from build123d import *

# Parameters (mm, degrees)
BOSS_EXTRUDE1_DEPTH = 36
CUT_EXTRUDE1_REACH  = 77.774
SKETCH5_W           = 10
SKETCH5_H           = 10
CUT_EXTRUDE4_DEPTH  = 70.808427336
SKETCH6_W           = 10
SKETCH6_H           = 49.869122111
CUT_EXTRUDE5_DEPTH  = 8.383745
SKETCH7_R           = 1.5
BOSS_EXTRUDE2_DEPTH = 10
BOSS_EXTRUDE3_DEPTH = 6
SKETCH9_R           = 5
BOSS_EXTRUDE4_DEPTH = 20.4
CUT_EXTRUDE7_REACH  = 76.44
SKETCH12_R          = 2
FILLET1_R           = 1.5


with BuildPart() as part:
    # Sketch1 → Boss-Extrude1 (new body)
    with BuildSketch(Plane.XY):
        Polygon((0, 0), (-26, 0), (-26, 10), (1.005154776, 56), (15.005154776, 56), align=None)
    extrude(amount=BOSS_EXTRUDE1_DEPTH)

    # Sketch2 → Cut-Extrude1 (cut, up to next)
    with BuildSketch(Plane(origin=(-26, 3.422964937, 0), x_dir=(0, 0, -1), z_dir=(1, 0, 0)), mode=Mode.PRIVATE) as cut_extrude1_sk1:
        with BuildLine():
            Line((-26, 36.577035063), (-26, 52.577035063))
            Line((-26, 52.577035063), (-36, 52.577035063))
            Line((-36, 52.577035063), (-36, 6.577035063))
            ThreePointArc((-36, 6.577035063), (-28.565835097, 20.765646762), (-26, 36.577035063))
        make_face()
    cut_extrude1_tool1 = extrude(cut_extrude1_sk1.sketch, amount=CUT_EXTRUDE1_REACH, mode=Mode.PRIVATE) & part.part
    # Sketch2 → Cut-Extrude1 (cut, up to next)
    with BuildSketch(Plane(origin=(-26, 3.422964937, 0), x_dir=(0, 0, -1), z_dir=(1, 0, 0)), mode=Mode.PRIVATE) as cut_extrude1_sk2:
        with BuildLine():
            ThreePointArc((-10, 36.577035063), (-7.434164903, 20.765646762), (0, 6.577035063))
            Line((0, 6.577035063), (0, 52.577035063))
            Line((0, 52.577035063), (-10, 52.577035063))
            Line((-10, 52.577035063), (-10, 36.577035063))
        make_face()
    cut_extrude1_tool2 = extrude(cut_extrude1_sk2.sketch, amount=CUT_EXTRUDE1_REACH, mode=Mode.PRIVATE) & part.part
    # Sketch2 → Cut-Extrude1 (cut, up to next)
    with BuildSketch(Plane(origin=(-26, 3.422964937, 0), x_dir=(0, 0, -1), z_dir=(1, 0, 0)), mode=Mode.PRIVATE) as cut_extrude1_sk3:
        with BuildLine():
            ThreePointArc((-36, 6.577035063), (-28.565835097, 20.765646762), (-26, 36.577035063))
            Line((-26, 36.577035063), (-26, 52.577035063))
            Line((-26, 52.577035063), (-36, 52.577035063))
            Line((-36, 52.577035063), (-36, 6.577035063))
        make_face()
    cut_extrude1_tool3 = extrude(cut_extrude1_sk3.sketch, amount=CUT_EXTRUDE1_REACH, mode=Mode.PRIVATE) & part.part
    # Sketch2 → Cut-Extrude1 (cut, up to next)
    with BuildSketch(Plane(origin=(-26, 3.422964937, 0), x_dir=(0, 0, -1), z_dir=(1, 0, 0)), mode=Mode.PRIVATE) as cut_extrude1_sk4:
        with BuildLine():
            Line((0, 6.577035063), (0, 52.577035063))
            Line((0, 52.577035063), (-10, 52.577035063))
            Line((-10, 52.577035063), (-10, 36.577035063))
            ThreePointArc((-10, 36.577035063), (-7.434164903, 20.765646762), (0, 6.577035063))
        make_face()
    cut_extrude1_tool4 = extrude(cut_extrude1_sk4.sketch, amount=CUT_EXTRUDE1_REACH, mode=Mode.PRIVATE) & part.part
    add(cut_extrude1_tool1.solids().sort_by_distance((-26, 37.109216, 31.540478))[0], mode=Mode.SUBTRACT)
    add(cut_extrude1_tool2.solids().sort_by_distance((-26, 37.109216, 4.459522))[0], mode=Mode.SUBTRACT)
    add(cut_extrude1_tool3.solids().sort_by_distance((-26, 37.109216, 31.540478))[0], mode=Mode.SUBTRACT)
    add(cut_extrude1_tool4.solids().sort_by_distance((-26, 37.109216, 4.459522))[0], mode=Mode.SUBTRACT)

    # Sketch5 → Cut-Extrude4 (cut, through all)
    with BuildSketch(Plane.ZY.offset(6)):
        with Locations((31, 5)):
            Rectangle(SKETCH5_W, SKETCH5_H)
        with Locations((5, 5)):
            Rectangle(SKETCH5_W, SKETCH5_H)
    extrude(amount=-CUT_EXTRUDE4_DEPTH, mode=Mode.SUBTRACT)

    # Sketch6 → Cut-Extrude5 (cut)
    with BuildSketch(Plane(origin=(0, 0, 0), x_dir=(0, 0, -1), z_dir=(0.9659258262890674, -0.2588190451025246, 0))):
        with Locations((-31, 33.040905048)):
            Rectangle(SKETCH6_W, SKETCH6_H)
        with Locations((-5, 33.040905048)):
            Rectangle(SKETCH6_W, SKETCH6_H)
    extrude(amount=-CUT_EXTRUDE5_DEPTH, mode=Mode.SUBTRACT)

    # Sketch7 → Boss-Extrude2 (add)
    with BuildSketch(Plane.XZ):
        Polygon((-26, 24), (-33, 34), (-33, 42), (-24, 42), (-24, 36), (-26, 36), align=None)
        with Locations(Location((-29.5, 37.5, 0), (0, 0, 270))):
            Circle(SKETCH7_R, mode=Mode.SUBTRACT)
        Polygon((-26, 0), (-24, 0), (-24, -6), (-33, -6), (-33, 2), (-26, 12), align=None)
        with Locations(Location((-29.5, -1.5, 0), (0, 0, 90))):
            Circle(SKETCH7_R, mode=Mode.SUBTRACT)
        Polygon((-6, 12), (1, 2), (1, -6), (-8, -6), (-8, 0), (-6, 0), align=None)
        with Locations(Location((-2.5, -1.5, 0), (0, 0, 270))):
            Circle(SKETCH7_R, mode=Mode.SUBTRACT)
        Polygon((-6, 36), (-8, 36), (-8, 42), (1, 42), (1, 34), (-6, 24), align=None)
        with Locations(Location((-2.5, 37.5, 0), (0, 0, 90))):
            Circle(SKETCH7_R, mode=Mode.SUBTRACT)
    extrude(amount=-BOSS_EXTRUDE2_DEPTH)

    # Sketch8 → Boss-Extrude3 (add, symmetric)
    with BuildSketch(Plane.XY.offset(18)):
        Polygon((-26, 5), (-26, 10), (0, 54.287840966), (0, 55.819136666), (-2, 55.819136666), (-27.5, 12.382984949), align=None)
    extrude(amount=BOSS_EXTRUDE3_DEPTH, both=True)

    # Sketch9 → Boss-Extrude4 (add)
    with BuildSketch(Plane(origin=(0, 0, 0), x_dir=(0, 0, -1), z_dir=(-0.9659258262890674, 0.2588190451025246, 0))):
        with Locations(Location((-18, -44.351999472, 0), (0, 0, 270))):
            Circle(SKETCH9_R)
    extrude(amount=BOSS_EXTRUDE4_DEPTH)

    # Sketch12 → Cut-Extrude7 (cut, up to next)
    with BuildSketch(Plane(origin=(-19.704886856, 5.27990852, 0), x_dir=(0, 0, 1), z_dir=(-0.9659258262890673, 0.2588190451025247, 0)), mode=Mode.PRIVATE) as cut_extrude7_sk1:
        with Locations(Location((18, 44.351999472, 0), (0, 0, 270))):
            Circle(SKETCH12_R)
    cut_extrude7_tool1 = extrude(cut_extrude7_sk1.sketch, amount=-CUT_EXTRUDE7_REACH, mode=Mode.PRIVATE) & part.part
    add(cut_extrude7_tool1.solids().sort_by_distance((-8.225745, 48.12065, 18))[0], mode=Mode.SUBTRACT)

    # Fillet1
    fillet1_edges = [part.edges().sort_by_distance(p)[0] for p in [
        (-28.5, 10, 42),
        (-28.5, 10, -6),
        (-3.5, 10, -6),
        (-3.5, 10, 42),
    ]]
    fillet(fillet1_edges, radius=FILLET1_R)


solid = part.part
Read the model definition and answer for the solid it produces. Units are mm, in the model's axes. A direction names the side the tool comes from. Round coordinates to 2 decimals unless told otherwise and drop trailing zeros. Order: outer loops, then holes, each group sorted by start corner. A loop starts at its lowest first (then second) coordinate and runs counter-clockwise, first axis right, second up.
1) Straight lines are drawn through the part: L1, parallel to X at y = 5.5, z = -1.5; L2, parallel to Z at x = -29, y = 6; L3, parallel to Z at x = -2, y = 4. For each, find the intervals that lie inside material, in ascending order.
2) Flat-ended cylindrical pins translate along their axes: pin 1 (2.5 mm diameter, centred on x = -2.5, z = 37.5, fed in from -Y); pin 2 (3 mm diameter, centred on x = -12, y = 12, fed in from +Z); pin 3 (4 mm diameter, centred on x = -20.5, z = 22.5, fed in from +Y); pin 4 (6.5 mm diameter, centred on y = 4, z = -1, fed in from +X). Find the tip coordinate at first contact, or state that the pin passes through.
3) For faces 1 (the face through (-1.84, 4.93, 6.06)), 2 (the face through (-26.76, 8.74, 18.08)), 3 (the face through (-28.44, 9.55, 41.57)), 4 (the face through (-28, 10, 2)), determine the directions among +Z, -Z, +X, -X, +Y, -Y from which every point of the face is accessible in a straight line to the end or side of a thin tool.
4) The part is cut by section A-A on x = -29.5. Write down the section's boundary in (y, z), plus the area to 3 significant figures.
5) The part is cut by section C-C on y = 7. Write down the section's boundary in (x, z).
6) The mould has two halves that part along Y. Classify faces 5 (the face through (-5.88, 52.43, 16.5)), 6 (the face through (-16, 5, 36)), 7 (the face through (-3.56, 9.57, -5.55)): released by +Y, released by -Y, zero draft, split by the parting line, or undercut.
7) The part is cut by section B-B on z = -1.5. Write down the section's boundary in (x, y).
8) The part is cut by section D-D on x = -22. Write down the section's boundary in (y, z).
Resolved:
1. L1: x = -33 to -31, -28 to -24, -8 to -4, -1 to 1
1. L2: z = -6 to -2.91, -0.09 to 7.71, 28.29 to 36.09, 38.91 to 42
1. L3: z = -6 to -2.91, -0.09 to 6.29, 10 to 26, 29.71 to 36.09, 38.91 to 42
2. pin 1: passes through
2. pin 2: stops at z = 35.63
2. pin 3: stops at y = 27.71
2. pin 4: stops at x = 1
3. face 1: +X, -Y
3. face 2: -X, -Y
3. face 3: +Z, +X, -X, +Y
3. face 4: -Z, -X, +Y
4. outline: (0, -6) - (8.5, -6) arc R1.5 ccw to (10, -4.5) - (10, -3) - (0, -3) - close; (0, 0) - (10, 0) - (10, 7) - (0, 7) - close; (0, 29) - (10, 29) - (10, 36) - (0, 36) - close; (0, 39) - (10, 39) - (10, 40.5) arc R1.5 ccw to (8.5, 42) - (0, 42) - close
4. area: 199 mm2
5. outline: (-33, -6) - (-24, -6) - (-24, 0) - (-8, 0) - (-8, -6) - (1, -6) - (1, 2) - (-4.6, 10) - (1.88, 10) - (1.88, 26) - (-4.6, 26) - (1, 34) - (1, 42) - (-8, 42) - (-8, 36) - (-24, 36) - (-24, 42) - (-33, 42) - (-33, 34) - (-26, 24) - (-26.41, 24) - (-26.41, 12) - (-26, 12) - (-33, 2) - close; hole circle Ø3 at (-29.5, -1.5); hole circle Ø3 at (-29.5, 37.5); hole circle Ø3 at (-2.5, -1.5); hole circle Ø3 at (-2.5, 37.5)
6. face 5: undercut
6. face 6: zero draft
6. face 7: released by +Y
7. outline: (-33, 0) - (-31, 0) - (-31, 10) - (-33, 10) - close; (-28, 0) - (-24, 0) - (-24, 10) - (-28, 10) - close; (-8, 0) - (-4, 0) - (-4, 10) - (-8, 10) - close; (-1, 0) - (1, 0) - (1, 10) - (-1, 10) - close
8. outline: (0, 0) - (10, 0) arc R50 cw to (16.81, 4.3) - (16.81, 12) - (21.75, 12) - (21.75, 24) - (16.81, 24) - (16.81, 31.7) arc R50 cw to (10, 36) - (0, 36) - close
